The listing builds one solid part. Answer for the finished solid, in the listing's coordinates (mm). Give positions to 0.01 mm unless a question says otherwise; leave off trailing zeros. Loops run counter-clockwise (first coordinate to the right, second up) from the corner with the lowest first, then second, coordinate; pieces in that order, holes last. Notation, with made-up numbers: (44.25, 67) -> (85.25, 67) arc R28 cw to (85.25, 92) -> close; hole circle Ø9 at (-12.5, -19.5). An arc over 180 degrees is marked (long way). One line per question, with ' | ' between items. Start each with the question number.
from build123d import *

# Parameters (mm, degrees)
SKETCH1_W                                      = 94
SKETCH1_H                                      = 23.2
BOSS_EXTRUDE1_DEPTH                            = 4
CHAMFER1_SIZE                                  = 5.5
CUT_EXTRUDE2_DEPTH                             = 48.12547082
CUT_EXTRUDE2_DEPTH_BACK                        = 48.12547082
SKETCH9_W                                      = 30.391833943
SKETCH9_H                                      = 23.2
SHELL1_START                                   = -9.1
SHELL1_DEPTH                                   = 18.2
FILLET1_R                                      = 1
M2_5X0_45_TAPPED_HOLE1_D                       = 2.05
M2_5X0_45_TAPPED_HOLE1_DEPTH                   = 6
M2_5X0_45_TAPPED_HOLE1_CSINK_D                 = 2.55
M2_5X0_45_TAPPED_HOLE1_CSINK_ANGLE             = 90
M2_5X0_45_TAPPED_HOLE1_TIP                     = 0.615882135
CSK_FOR_M2_5_FLAT_HEAD_MACHINE_SCREW1_AT_COUNT = 2
CSK_FOR_M2_5_FLAT_HEAD_MACHINE_SCREW1_AT_PITCH = 8.544003745
CSK_FOR_M2_5_FLAT_HEAD_MACHINE_SCREW_2_COUNT   = 2
CSK_FOR_M2_5_FLAT_HEAD_MACHINE_SCREW_2_PITCH   = 10.307764064
SKETCH8_W                                      = 19.75
SKETCH8_H                                      = 5.25
CUT_EXTRUDE1_DEPTH                             = 47.042073151
FILLET5_R                                      = 1
FILLET5_OF_MIRROR1_R                           = 1


# Read off the part's stored shape, not the designer's step: Shell1
with BuildPart() as part:
    # Sketch1 → Boss-Extrude1 (new body)
    with BuildSketch(Plane.XY):
        Rectangle(SKETCH1_W, SKETCH1_H)
    extrude(amount=BOSS_EXTRUDE1_DEPTH)

    # Chamfer1
    # the kernel refuses this chamfer: 5.5 mm, written as the material it takes off along each edge
    with BuildSketch(Plane(origin=(47, 25.744256434, 0), x_dir=(0.027495876610585942, 0, 0.9996219169112968), z_dir=(0, -1, 0)), Plane(origin=(-47, -25.744256434, 0), x_dir=(-0.027495876610585942, 0, 0.9996219169112968), z_dir=(0, 1, 0))) as chamfer1_piece_1:
        Polygon((CHAMFER1_SIZE * 0.999621916911, CHAMFER1_SIZE * 0.0274958766106), (-CHAMFER1_SIZE * 0.0274958766106, CHAMFER1_SIZE * 0.999621916911), (0, 0), align=None)
    extrude(amount=51.488512868, mode=Mode.SUBTRACT)

    # Sketch9 → Cut-Extrude2 (cut, two sides: drawn at the far end of the back side and taken through both)
    with BuildSketch(Plane(origin=(0, 0, 0), x_dir=(-1, 0, 0), z_dir=(0, 0, -1)).offset(-CUT_EXTRUDE2_DEPTH_BACK)):
        with Locations((-59.695916972, 0)):
            Rectangle(SKETCH9_W, SKETCH9_H)
        with Locations((59.695916972, 0)):
            Rectangle(SKETCH9_W, SKETCH9_H)
    extrude(amount=CUT_EXTRUDE2_DEPTH + CUT_EXTRUDE2_DEPTH_BACK, mode=Mode.SUBTRACT)

    # Shell1 outline → Shell1 (cut)
    with BuildSketch(Plane(origin=(0, 0, 0), x_dir=(1, 0, 0), z_dir=(0, 1, 0)).offset(SHELL1_START)):
        Polygon((-41.5, 0), (-43.75, -2.25), (43.75, -2.25), (41.5, 0), align=None)
    extrude(amount=SHELL1_DEPTH, mode=Mode.SUBTRACT)

    # Fillet1
    fillet1_edges = [part.edges().sort_by_distance(p)[0] for p in [
        (0, 9.1, 2.25),
        (0, -9.1, 2.25),
    ]]
    fillet(fillet1_edges, radius=FILLET1_R)

    # M2.5x0.45 Tapped Hole1
    with Locations(Plane(origin=(0, 0, 2.25), x_dir=(-1, 0, 0), z_dir=(0, 0, -1))):
        with Locations((0, 2.6), (-22, 6.6), (-22, -1.4), (22, -1.4), (22, 6.6)):
            CounterSinkHole(M2_5X0_45_TAPPED_HOLE1_D / 2, M2_5X0_45_TAPPED_HOLE1_CSINK_D / 2, depth=M2_5X0_45_TAPPED_HOLE1_DEPTH, counter_sink_angle=M2_5X0_45_TAPPED_HOLE1_CSINK_ANGLE)
            with Locations((0, 0, -(M2_5X0_45_TAPPED_HOLE1_DEPTH + M2_5X0_45_TAPPED_HOLE1_TIP / 2))):  # 118° drill point
                Cone(0, M2_5X0_45_TAPPED_HOLE1_D / 2, M2_5X0_45_TAPPED_HOLE1_TIP, mode=Mode.SUBTRACT)

    # Sketch5 → CSK for M2.5 Flat Head Machine Screw1 (revolve, cut)
    with BuildSketch(Plane(origin=(36, -1.1, 2.25), x_dir=(0, 1, 0), z_dir=(1, 0, 0))):
        Polygon((0, 0), (0, 7.321247898), (1.45, 6.45), (1.45, 1.3), (2.75, 0), align=None)
    csk_for_m2_5_flat_head_machine_screw1 = revolve(axis=Axis((36, -1.1, -4.1), (0, 0, 1)), mode=Mode.SUBTRACT)

    # CSK for M2.5 Flat Head Machine Screw1 at: CSK for M2.5 Flat Head Machine Screw1 ×2
    with Locations(*[Vector(0.35112344158839104, -0.9363291775690448, 0) * (i * CSK_FOR_M2_5_FLAT_HEAD_MACHINE_SCREW1_AT_PITCH) for i in range(1, CSK_FOR_M2_5_FLAT_HEAD_MACHINE_SCREW1_AT_COUNT)]):
        add(csk_for_m2_5_flat_head_machine_screw1, mode=Mode.SUBTRACT)

    # CSK for M2.5 Flat Head Machine Screw 2: CSK for M2.5 Flat Head Machine Screw1 ×2
    with Locations(*[Vector(-0.6305926250944661, -0.7761140001162652, 0) * (i * CSK_FOR_M2_5_FLAT_HEAD_MACHINE_SCREW_2_PITCH) for i in range(1, CSK_FOR_M2_5_FLAT_HEAD_MACHINE_SCREW_2_COUNT)]):
        add(csk_for_m2_5_flat_head_machine_screw1, mode=Mode.SUBTRACT)

    # Sketch8 → Cut-Extrude1 (cut, through all)
    with BuildSketch(Plane(origin=(0, 0, 2.25), x_dir=(-1, 0, 0), z_dir=(0, 0, -1))):
        with Locations((-34.625, -8.975)):
            Rectangle(SKETCH8_W, SKETCH8_H)
    cut_extrude1 = extrude(amount=CUT_EXTRUDE1_DEPTH, mode=Mode.SUBTRACT)

    # Fillet5
    fillet5_edges = [part.edges().sort_by_distance(p)[0] for p in [
        (24.75, -9.85, 2.25),
    ]]
    fillet(fillet5_edges, radius=FILLET5_R)

    # Mirror1: CSK for M2.5 Flat Head Machine Screw1, Cut-Extrude1 across plane
    add(csk_for_m2_5_flat_head_machine_screw1.mirror(Plane(origin=(0, 0, 0), x_dir=(0, 0, 1), z_dir=(1, 0, 0))), mode=Mode.SUBTRACT)
    add(cut_extrude1.mirror(Plane(origin=(0, 0, 0), x_dir=(0, 0, 1), z_dir=(1, 0, 0))), mode=Mode.SUBTRACT)

    # Mirror1 copy 1 sketch → Mirror1 copy 1 (revolve, cut)
    with BuildSketch(Plane(origin=(-39, -9.1, 2.25), x_dir=(0, 1, 0), z_dir=(-1, 0, 0))):
        Polygon((0, 0), (0, -7.321247898), (1.45, -6.45), (1.45, -1.3), (2.75, 0), align=None)
    revolve(axis=Axis((-39, -9.1, -4.1), (0, 0, -1)), mode=Mode.SUBTRACT)

    # Mirror1 copy 2 sketch → Mirror1 copy 2 (revolve, cut)
    with BuildSketch(Plane(origin=(-29.5, -9.1, 2.25), x_dir=(0, 1, 0), z_dir=(-1, 0, 0))):
        Polygon((0, 0), (0, -7.321247898), (1.45, -6.45), (1.45, -1.3), (2.75, 0), align=None)
    revolve(axis=Axis((-29.5, -9.1, -4.1), (0, 0, -1)), mode=Mode.SUBTRACT)

    # Fillet5 of Mirror1
    fillet5_of_mirror1_edges = [part.edges().sort_by_distance(p)[0] for p in [
        (-24.75, -9.85, 2.25),
    ]]
    fillet(fillet5_of_mirror1_edges, radius=FILLET5_OF_MIRROR1_R)


solid = part.part
1. The part is cut by section D-D (x = -14). Write down the section's boundary in (y, z).
2. Each of these flat-tipped pins is pushed along its axis until it touches: pin 1 Ø4.5 at (x, y) = (-39, -9.1) entering from -Z; pin 2 Ø1 at (y, z) = (-10.5, 0.5) entering from -X; pin 3 Ø5 at (x, y) = (-31.5, 3.5) entering from -Z. Where does it stop, or does it pass through?
3. Straight lines are drawn through the part: L1, parallel to Y at x = 22, z = 3.2 (3 decimals); L2, parallel to X at y = 6.6, z = 3.3 (3 decimals); L3, parallel to Y at x = -3, z = 0.95. For each, find the intervals that lie inside material, in ascending order.
4. The part is cut by section B-B (y = 2.6). Write down the section's boundary in (x, z) (3 decimals).
5. The part is cut by section A-A (x = -29.5). Write down the section's boundary in (y, z).
6. Determine the mould class of faces 1 (the conical face through (-34, -1, 3)), 2 (the flat face through (-43.9, 2.5, 2.4)), 3 (the flat face through (-1, 0, 2.25)), 4 (the cylindrical face through (-0.133, 3.616, 3.26)) for opening direction X: released by +X, released by -X, zero draft, split by the parting line, or undercut.
7. The part is cut by section C-C (x = 22). Write down the section's boundary in (y, z) (3 decimals).
Check sheet entries:
1) outline: (-11.6, 0) -> (-9.1, 0) -> (-9.1, 1.25) arc R1 cw to (-8.1, 2.25) -> (8.1, 2.25) arc R1 cw to (9.1, 1.25) -> (9.1, 0) -> (11.6, 0) -> (11.6, 4) -> (-11.6, 4) -> close
2) pin 1: stops at z = 2.75 | pin 2: stops at x = -24.75 | pin 3: stops at z = 2.25
3) L1: y = -11.6 to -2.425, -0.375 to 5.575, 7.625 to 11.6 | L2: x = -44.5 to -23.025, -20.975 to 20.975, 23.025 to 44.5 | L3: y = -11.6 to -9.1, 9.1 to 11.6
4) outline: (-44.5, 3) -> (-43.75, 2.25) -> (-1.275, 2.25) -> (-1.025, 2.5) -> (-1.025, 4) -> (-44.5, 4) -> close; (1.025, 2.5) -> (1.275, 2.25) -> (43.75, 2.25) -> (44.5, 3) -> (44.5, 4) -> (1.025, 4) -> close
5) outline: (-11.6, 2.5) -> (-10.55, 3.55) -> (-10.55, 4) -> (-11.6, 4) -> close; (-7.65, 3.55) -> (-6.35, 2.25) -> (8.1, 2.25) arc R1 cw to (9.1, 1.25) -> (9.1, 0) -> (11.6, 0) -> (11.6, 4) -> (-7.65, 4) -> close
6) face 1: undercut | face 2: released by -X | face 3: zero draft | face 4: undercut
7) outline: (-11.6, 0) -> (-9.1, 0) -> (-9.1, 1.25) arc R1 cw to (-8.1, 2.25) -> (-2.675, 2.25) -> (-2.425, 2.5) -> (-2.425, 4) -> (-11.6, 4) -> close; (-0.375, 2.5) -> (-0.125, 2.25) -> (5.325, 2.25) -> (5.575, 2.5) -> (5.575, 4) -> (-0.375, 4) -> close; (7.625, 2.5) -> (7.875, 2.25) -> (8.1, 2.25) arc R1 cw to (9.1, 1.25) -> (9.1, 0) -> (11.6, 0) -> (11.6, 4) -> (7.625, 4) -> close
